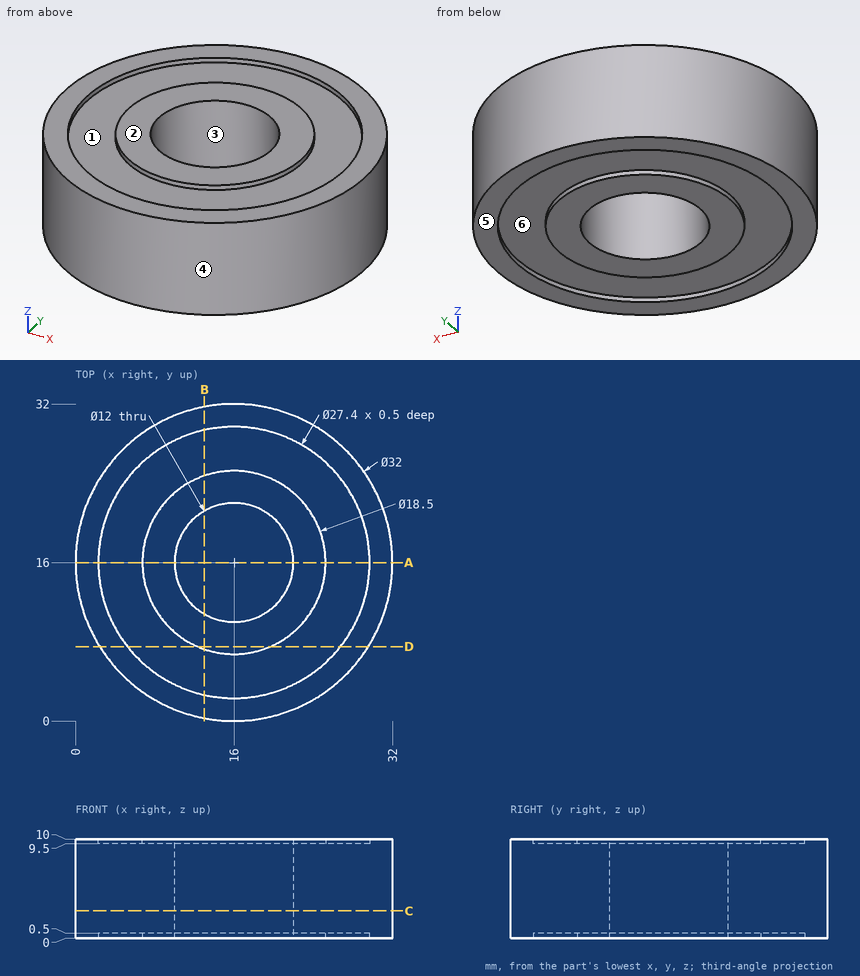
Here's the drawing with two shaded views (mm, measured from the low corner). I have some questions. A direction names the side the tool comes from. Give positions to 0.01 mm unless a question says otherwise; leave off trailing zeros. Order: outer loops, then holes, each group sorted by start corner. A loop starts at its lowest first (then second) coordinate and runs counter-clockwise, first axis right, second up. Notation, with made-up numbers: (-24, 46.25) -> (-17, 46.25) arc R11 ccw to (-17, 51.25) -> close; hole circle Ø4 at (42.5, 27). An arc over 180 degrees is marked (long way). Use a Markdown table: item, result. Add a question column.
Item 1: Will these pins go through, and if not, where does the flat tip stop? pin 1 (19 mm diameter, centred on x = 16, y = 16, fed in from -Z); pin 2 (3 mm diameter, centred on y = 11.5, z = 6, fed in from -X); pin 3 (4 mm diameter, centred on y = 26, z = 4, fed in from +X); pin 4 (3 mm diameter, centred on x = 10, y = 25, fed in from -Z).
Item 2: Imagine slicing it at C-C on z = 2.75. Please give me the cut outline in (x, y), plus the area to 3 significant figures.
Item 3: I need wall thicknesses on line 1 (Y direction, x = 16, z = 6.5); line 2 (Z direction, x = 5, y = 8); line 3 (Y direction, x = 13.5, z = 3.75). Which ranges of each line are inside material? Lowest first, please.
Item 4: For the marked faces 5 and 6, which set-ups out of +Z, -Z, +X, -X, +Y, -Y let a thin tool reach every point of the face, with its end or its side?
Item 5: Imagine slicing it at D-D on y = 7.5. Please give me the cut outline in (x, z).
Item 6: Imagine slicing it at A-A on y = 16. Please give me the cut outline in (x, z), plus the area to 3 significant figures.
Item 7: Imagine slicing it at B-B on x = 13. Please give me the cut outline in (y, z).
Item 8: If we mould it in two halves opening along Y, with no side actions, what happens to the marked faces 1, 2, 3 and 4? For each: pulls with the +Y half, pulls with the -Y half, needs draft (parallel to the pull), parting line crosses it, or undercut.
Data:
| question | item | result |
|---|---|---|
| 1 | pin 1 | stops at z = 0 |
| 1 | pin 2 | stops at x = 0.28 |
| 1 | pin 3 | stops at x = 29.86 |
| 1 | pin 4 | stops at z = 0.5 |
| 2 | outline | circle Ø32 at (16, 16); hole circle Ø12 at (16, 16) |
| 2 | area | 691 mm² |
| 3 | line 1 | y = 0 to 10, 22 to 32 |
| 3 | line 2 | z = 0.5 to 9.5 |
| 3 | line 3 | y = 0.2 to 10.55, 21.45 to 31.8 |
| 4 | face 5 | -Z, +X, -X, +Y, -Y |
| 4 | face 6 | -Z |
| 5 | outline | (2.44, 0) -> (5.26, 0) -> (5.26, 0.5) -> (12.35, 0.5) -> (12.35, 0) -> (19.65, 0) -> (19.65, 0.5) -> (26.74, 0.5) -> (26.74, 0) -> (29.56, 0) -> (29.56, 10) -> (26.74, 10) -> (26.74, 9.5) -> (19.65, 9.5) -> (19.65, 10) -> (12.35, 10) -> (12.35, 9.5) -> (5.26, 9.5) -> (5.26, 10) -> (2.44, 10) -> close |
| 6 | outline | (0, 0) -> (2.3, 0) -> (2.3, 0.5) -> (6.75, 0.5) -> (6.75, 0) -> (10, 0) -> (10, 10) -> (6.75, 10) -> (6.75, 9.5) -> (2.3, 9.5) -> (2.3, 10) -> (0, 10) -> close; (22, 0) -> (25.25, 0) -> (25.25, 0.5) -> (29.7, 0.5) -> (29.7, 0) -> (32, 0) -> (32, 10) -> (29.7, 10) -> (29.7, 9.5) -> (25.25, 9.5) -> (25.25, 10) -> (22, 10) -> close |
| 6 | area | 191 mm² |
| 7 | outline | (0.28, 0) -> (2.63, 0) -> (2.63, 0.5) -> (7.25, 0.5) -> (7.25, 0) -> (10.8, 0) -> (10.8, 10) -> (7.25, 10) -> (7.25, 9.5) -> (2.63, 9.5) -> (2.63, 10) -> (0.28, 10) -> close; (21.2, 0) -> (24.75, 0) -> (24.75, 0.5) -> (29.37, 0.5) -> (29.37, 0) -> (31.72, 0) -> (31.72, 10) -> (29.37, 10) -> (29.37, 9.5) -> (24.75, 9.5) -> (24.75, 10) -> (21.2, 10) -> close |
| 8 | face 1 | undercut |
| 8 | face 2 | needs draft |
| 8 | face 3 | undercut |
| 8 | face 4 | parting line crosses it |
